Autodesk Inventor part; units mm, degrees
ref_plane "YZ Plane" through (0, 0, 0) normal (1, 0, 0) x (0, 1, 0)
ref_plane "XZ Plane" through (0, 0, 0) normal (0, 1, 0) x (-1, 0, 0)
ref_plane "XY Plane" through (0, 0, 0) normal (0, 0, 1) x (1, 0, 0)
sketch "Sketch1" plane through (0, 0, 0) normal (0, 1, 0) x (-1, 0, 0)
  line L0 (0, 0) -> (508, 0)
  line L1 (508, 0) -> (508, -381)
  line L2 (508, -381) -> (0, -381)
  line L3 (0, -381) -> (0, 0)
  line L4 (0, 0) -> (50.8, 0)
  line L5 (0, 0) -> (0, -12.7)
  line L6 (0, -6.35) -> (0, -57.1551)
  line L7 (0, -6.35) -> (50.8, -6.35)
  line L8 (50.8, -6.35) -> (50.8, -57.1551)
  line L9 (50.8, -57.1551) -> (0, -57.1551)
  line L10 (0, -57.1551) -> (0, -6.35)
  line L11 (0, -57.1551) -> (0, -66.0049)
  line L12 (0, -57.1551) -> (0, -69.8551)
  line L13 (0, -57.1551) -> (0, -63.5051)
  line L14 (0, -63.5051) -> (0, -317.5051)
  line L15 (0, -63.5051) -> (50.8, -63.5051)
  line L16 (50.8, -63.5051) -> (50.8, -317.5051)
  line L17 (50.8, -317.5051) -> (0, -317.5051)
  line L18 (0, -317.5051) -> (0, -63.5051)
  line L19 (0, -381) -> (0, -374.6428)
  line L20 (0, -317.5051) -> (0, -323.8478)
  line L21 (0, -323.8478) -> (50.8, -323.8478)
  line L22 (50.8, -323.8478) -> (50.8, -374.6428)
  line L23 (50.8, -374.6428) -> (0, -374.6428)
  line L24 (0, -374.6428) -> (0, -323.8478)
  line L25 (508, 0) -> (457.2, 0)
  line L26 (508, -6.35) -> (457.2, -6.35)
  line L27 (457.2, -6.35) -> (457.2, -57.1551)
  line L28 (457.2, -57.1551) -> (508, -57.1551)
  line L29 (508, -57.1551) -> (508, -6.35)
  line L30 (508, -63.5051) -> (457.2, -63.5051)
  line L31 (457.2, -63.5051) -> (457.2, -317.5051)
  line L32 (457.2, -317.5051) -> (508, -317.5051)
  line L33 (508, -317.5051) -> (508, -63.5051)
  line L34 (508, -323.8478) -> (457.2, -323.8478)
  line L35 (457.2, -323.8478) -> (457.2, -374.6428)
  line L36 (457.2, -374.6428) -> (508, -374.6428)
  line L37 (508, -374.6428) -> (508, -323.8478)
  line L38 (508, 0) -> (533.4, 0)
  line L39 (533.4, 0) -> (533.4, 25.4)
  line L40 (0, -381) -> (-25.4, -381)
  line L41 (-25.4, -381) -> (-25.4, -406.4)
  line L42 (533.4, 25.4) -> (-25.4, 25.4)
  line L43 (-25.4, 25.4) -> (-25.4, -406.4)
  line L44 (-25.4, -406.4) -> (533.4, -406.4)
  line L45 (533.4, -406.4) -> (533.4, 25.4)
extrude "Extrusion1" add sketch "Sketch1" along normal blind 254 contours L3 L40 L43 L42 L39 L38 L0 | L38 L45 L44 L41 L40 L2 L1
extrude "Extrusion2" add sketch "Sketch1" along normal blind 127 contours L0 L1 L26 L27 L28 L30 L31 L32 L34 L35 L36 L2 L3 L23 L22 L21 L17 L16 L15 L9 L8 L7
extrude "Extrusion3" add sketch "Sketch1" along normal blind 127 contours L7 L8 L9 L3 | L1 L28 L27 L26 | L1 L36 L35 L34 | L21 L22 L23 L3
extrude "Extrusion4" add sketch "Sketch1" along normal blind 38.1 contours L15 L16 L17 L3 | L1 L32 L31 L30
sketch "Sketch2" plane through (25.4, 0, 25.4) normal (1, 0, 0) x (0, 0, -1)
  line L0 (342.9051, 38.1) -> (88.9051, 38.1)
  line L1 (88.9051, 38.1) -> (88.9051, 63.5)
  line L2 (88.9051, 127) -> (88.9051, 38.1)
  line L3 (88.9051, 63.5) -> (342.9051, 63.5)
  line L4 (342.9051, 63.5) -> (342.9051, 38.1)
  line L5 (342.9051, 38.1) -> (88.9051, 38.1)
  line L6 (88.9051, 38.1) -> (88.9051, 63.5)
  point P0 (25.4, 0)
  dimension "d21" = 25.4
extrude "Extrusion5" cut sketch "Sketch2" against normal blind 76.2
sketch "Sketch3" plane through (-533.4, 0, -406.4) normal (-1, 0, 0) x (0, 0, 1)
  line L0 (88.8949, 63.5) -> (88.8949, 38.1)
  line L1 (342.8949, 38.1) -> (342.8949, 127)
  line L2 (88.8949, 63.5) -> (342.8949, 63.5)
  line L3 (342.8949, 63.5) -> (342.8949, 38.1)
  line L4 (342.8949, 38.1) -> (88.8949, 38.1)
  line L5 (88.8949, 38.1) -> (88.8949, 63.5)
  point P0 (406.4, 0)
extrude "Extrusion6" cut sketch "Sketch3" against normal blind 76.2
properties part number "Board"
Design review of the part built by this model. Coordinates are the model's own, in mm. A direction names the side the tool comes from. Coordinates: 2 decimals unless noted, no trailing zeros. Order: outer loops, then holes, each group sorted by start corner. A loop starts at its lowest first (then second) coordinate and runs counter-clockwise, first axis right, second up.
Item 1: The part is to be moulded in two halves that separate along Z. For faces 6 (the flat face through (-533.4, 125, -194)), 7 (the flat face through (-12, 38.1, -192)), 8 (the flat face through (-258, 125, 25.4)), say which applies: pulls with the +Z half, pulls with the -Z half, needs draft (parallel to the pull), parting line crosses it, or undercut.
Item 2: Take a section at C-C, the plane y = 72. Write out the cut boundary in (x, z).
Item 3: Take a section at D-D, the plane x = -330.5. Write out the cut boundary in (y, z), then the cut area to 3 significant figures.
Item 4: For pin 1 Ø10 at (x, z) = (-239, -271.5) entering from +Y, flat-tipped, find the tip position at first contact; note if it passes through.
Item 5: Take a section at A-A, the plane y = 133.5. Write out the cut boundary in (x, z).
Item 6: For line 1 (X direction, y = 104.5, z = -76.5); line 2 (Z direction, x = -327, y = 142); line 3 (X direction, y = 229, z = -176), list the stretches that pass through material, from the lowest coordinate up.
Item 7: Take a section at B-B, the plane z = -237. Write out the cut boundary in (x, y), then the cut area to 3 significant figures.
Item 8: For faces 1 (the flat face through (-250, 125, -406.4)), 2 (the flat face through (-521, 63.5, -192)), 3 (the flat face through (-250, 190, 0)), 4 (the flat face through (-487, 82, -63.505)), 5 (the flat face through (13, 63.5, -189)), list the 3-axis set-ups (+Z, -Z, +X, -X, +Y, -Y) from which the entire face can be reached by the end or side of a thin tool; tool diameter is ignored.
The answers:
1. face 6: needs draft
1. face 7: undercut
1. face 8: pulls with the +Z half
2. outline: (-533.4, -406.4) - (25.4, -406.4) - (25.4, 25.4) - (-533.4, 25.4) - close; hole (-508, -317.51) - (-457.2, -317.51) - (-457.2, -63.51) - (-508, -63.51) - close; hole (-50.8, -317.51) - (0, -317.51) - (0, -63.51) - (-50.8, -63.51) - close
3. outline: (0, -406.4) - (254, -406.4) - (254, -381) - (127, -381) - (127, 0) - (254, 0) - (254, 25.4) - (0, 25.4) - close
3. area: 61,300 mm2
4. pin 1: stops at y = 127
5. outline: (-533.4, -406.4) - (25.4, -406.4) - (25.4, 25.4) - (-533.4, 25.4) - close; hole (-508, -381) - (0, -381) - (0, 0) - (-508, 0) - close
6. line 1: x = -533.4 to -508, -457.2 to -50.8, 0 to 25.4
6. line 2: z = -406.4 to -381, 0 to 25.4
6. line 3: x = -533.4 to -508, 0 to 25.4
7. outline: (-533.4, 0) - (25.4, 0) - (25.4, 38.1) - (-50.8, 38.1) - (-50.8, 127) - (-457.2, 127) - (-457.2, 38.1) - (-533.4, 38.1) - close; (-533.4, 63.5) - (-508, 63.5) - (-508, 254) - (-533.4, 254) - close; (0, 63.5) - (25.4, 63.5) - (25.4, 254) - (0, 254) - close
7. area: 67,100 mm2
8. face 1: -Z, +X, -X, +Y, -Y
8. face 2: -X
8. face 3: +Y
8. face 4: none
8. face 5: +X
